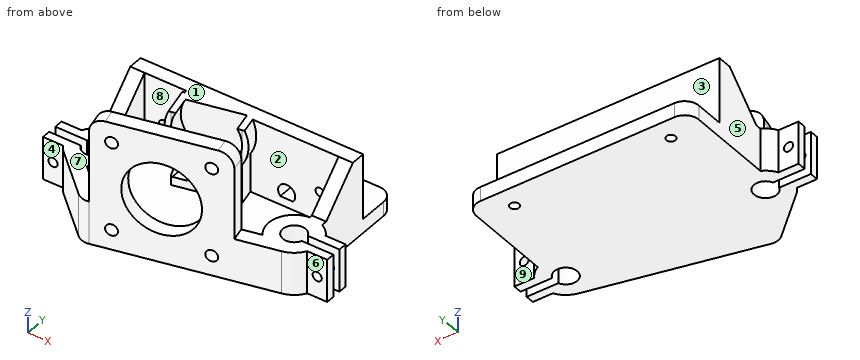
from build123d import *

# Parameters (mm, degrees)
BOSS_EXTRUDE1_DEPTH = 15
SKETCH2_R           = 1.6
CUT_EXTRUDE1_DEPTH  = 62.324670446
BOSS_EXTRUDE2_DEPTH = 30
FILLET1_R           = 5
CUT_EXTRUDE2_REACH  = 84.635
SKETCH4_R           = 12.5
SKETCH4_R_2         = 2
BOSS_EXTRUDE3_DEPTH = 2
BOSS_EXTRUDE4_DEPTH = 26
SKETCH7_W           = 78
SKETCH7_H           = 13
BOSS_EXTRUDE5_DEPTH = 5
BOSS_EXTRUDE6_DEPTH = 10
SKETCH9_R           = 11
CUT_EXTRUDE4_DEPTH  = 7
CHAMFER1_SIZE       = 13
SKETCH10_W          = 78
SKETCH10_H          = 5
BOSS_EXTRUDE7_DEPTH = 15
SKETCH11_R          = 1.6
CUT_EXTRUDE5_DEPTH  = 77.996527229
CUT_EXTRUDE6_REACH  = 85.597
SKETCH12_R          = 1.5
FILLET2_R           = 5
CUT_EXTRUDE7_REACH  = 85.597


with BuildPart() as part:
    # Sketch1 → Boss-Extrude1 (new body)
    with BuildSketch(Plane.XY):
        with BuildLine():
            Line((-39, 28), (39, 28))
            Line((39, 28), (39, 8.062257748))
            ThreePointArc((39, 8.062257748), (41.160225429, 6.561373535), (42.794228634, 4.5))
            Line((42.794228634, 4.5), (49.794228634, 4.5))
            Line((49.794228634, 4.5), (49.794228634, 1.5))
            Line((49.794228634, 1.5), (38.708099244, 1.5))
            ThreePointArc((38.708099244, 1.5), (31, 0), (38.708099244, -1.5))
            Line((38.708099244, -1.5), (49.794228634, -1.5))
            Line((49.794228634, -1.5), (49.794228634, -4.5))
            Line((49.794228634, -4.5), (42.794228634, -4.5))
            ThreePointArc((42.794228634, -4.5), (40.323053514, -7.257072501), (36.951023531, -8.785983564))
            Line((36.951023531, -8.785983564), (-23.82345919, -22.281620679))
            Line((-23.82345919, -22.281620679), (-41.045145267, -6.667549678))
            ThreePointArc((-41.045145267, -6.667549678), (-42.004044217, -5.651846124), (-42.794228634, -4.5))
            Line((-42.794228634, -4.5), (-49.794228634, -4.5))
            Line((-49.794228634, -4.5), (-49.794228634, -1.5))
            Line((-49.794228634, -1.5), (-38.708099244, -1.5))
            ThreePointArc((-38.708099244, -1.5), (-31, 0), (-38.708099244, 1.5))
            Line((-38.708099244, 1.5), (-49.794228634, 1.5))
            Line((-49.794228634, 1.5), (-49.794228634, 4.5))
            Line((-49.794228634, 4.5), (-42.794228634, 4.5))
            ThreePointArc((-42.794228634, 4.5), (-41.160225429, 6.561373535), (-39, 8.062257748))
            Line((-39, 8.062257748), (-39, 28))
        make_face()
        with BuildLine():
            Line((-34, 23), (34, 23))
            Line((34, 23), (34, 8.94427191))
            ThreePointArc((34, 8.94427191), (26.676479172, 3.423302649), (27.996581118, -5.652620982))
            Line((27.996581118, -5.652620982), (-22.38171768, -16.839672004))
            Line((-22.38171768, -16.839672004), (-31.713897446, -8.378635331))
            ThreePointArc((-31.713897446, -8.378635331), (-26.077363193, 1.177519599), (-34, 8.94427191))
            Line((-34, 8.94427191), (-34, 23))
        make_face(mode=Mode.SUBTRACT)
    extrude(amount=BOSS_EXTRUDE1_DEPTH)

    # Sketch2 → Cut-Extrude1 (cut, through all)
    with BuildSketch(Plane.XZ.offset(4.5)):
        with Locations((-46.294228634, 7.5)):
            Circle(SKETCH2_R)
        with Locations((46.294228634, 7.5)):
            Circle(SKETCH2_R)
    extrude(amount=-CUT_EXTRUDE1_DEPTH, mode=Mode.SUBTRACT)

    # Sketch3 → Boss-Extrude2 (add)
    with BuildSketch(Plane.XY.offset(15)):
        Polygon((-22.38171768, -16.839672004), (-21.297815718, -21.720773984), (22.6321021, -11.965656329), (21.548200138, -7.084554349), align=None)
    extrude(amount=BOSS_EXTRUDE2_DEPTH)

    # Fillet1
    fillet1_edges = [part.edges().sort_by_distance(p)[0] for p in [
        (-23.82345919, -22.281620679, 7.5),
        (22.090151119, -9.525105339, 45),
        (-21.839766699, -19.280222994, 45),
    ]]
    fillet(fillet1_edges, radius=FILLET1_R)

    # Sketch4 → Cut-Extrude2 (cut, up to next)
    with BuildSketch(Plane(origin=(3.595804379, -16.192873979, 0), x_dir=(0.9762203959642155, 0.21678039234089044, 0), z_dir=(0.21678039234089044, -0.9762203959642155, 0)), mode=Mode.PRIVATE) as cut_extrude2_sk1:
        with Locations((-3, 22.5)):
            Circle(SKETCH4_R)
    cut_extrude2_tool1 = extrude(cut_extrude2_sk1.sketch, amount=-CUT_EXTRUDE2_REACH, mode=Mode.PRIVATE) & part.part
    # Sketch4 → Cut-Extrude2 (cut, up to next)
    with BuildSketch(Plane(origin=(3.595804379, -16.192873979, 0), x_dir=(0.9762203959642155, 0.21678039234089044, 0), z_dir=(0.21678039234089044, -0.9762203959642155, 0)), mode=Mode.PRIVATE) as cut_extrude2_sk2:
        with Locations((-18.5, 38)):
            Circle(SKETCH4_R_2)
    cut_extrude2_tool2 = extrude(cut_extrude2_sk2.sketch, amount=-CUT_EXTRUDE2_REACH, mode=Mode.PRIVATE) & part.part
    # Sketch4 → Cut-Extrude2 (cut, up to next)
    with BuildSketch(Plane(origin=(3.595804379, -16.192873979, 0), x_dir=(0.9762203959642155, 0.21678039234089044, 0), z_dir=(0.21678039234089044, -0.9762203959642155, 0)), mode=Mode.PRIVATE) as cut_extrude2_sk3:
        with Locations((12.5, 38)):
            Circle(SKETCH4_R_2)
    cut_extrude2_tool3 = extrude(cut_extrude2_sk3.sketch, amount=-CUT_EXTRUDE2_REACH, mode=Mode.PRIVATE) & part.part
    # Sketch4 → Cut-Extrude2 (cut, up to next)
    with BuildSketch(Plane(origin=(3.595804379, -16.192873979, 0), x_dir=(0.9762203959642155, 0.21678039234089044, 0), z_dir=(0.21678039234089044, -0.9762203959642155, 0)), mode=Mode.PRIVATE) as cut_extrude2_sk4:
        with Locations((12.5, 7)):
            Circle(SKETCH4_R_2)
    cut_extrude2_tool4 = extrude(cut_extrude2_sk4.sketch, amount=-CUT_EXTRUDE2_REACH, mode=Mode.PRIVATE) & part.part
    # Sketch4 → Cut-Extrude2 (cut, up to next)
    with BuildSketch(Plane(origin=(3.595804379, -16.192873979, 0), x_dir=(0.9762203959642155, 0.21678039234089044, 0), z_dir=(0.21678039234089044, -0.9762203959642155, 0)), mode=Mode.PRIVATE) as cut_extrude2_sk5:
        with Locations((-18.5, 7)):
            Circle(SKETCH4_R_2)
    cut_extrude2_tool5 = extrude(cut_extrude2_sk5.sketch, amount=-CUT_EXTRUDE2_REACH, mode=Mode.PRIVATE) & part.part
    add(cut_extrude2_tool1.solids().sort_by_distance((0.667143, -16.843215, 22.5))[0], mode=Mode.SUBTRACT)
    add(cut_extrude2_tool2.solids().sort_by_distance((-14.464273, -20.203311, 38))[0], mode=Mode.SUBTRACT)
    add(cut_extrude2_tool3.solids().sort_by_distance((15.798559, -13.483119, 38))[0], mode=Mode.SUBTRACT)
    add(cut_extrude2_tool4.solids().sort_by_distance((15.798559, -13.483119, 7))[0], mode=Mode.SUBTRACT)
    add(cut_extrude2_tool5.solids().sort_by_distance((-14.464273, -20.203311, 7))[0], mode=Mode.SUBTRACT)

    # Sketch5 → Boss-Extrude3 (add)
    with BuildSketch(Plane(origin=(0, 0, 0), x_dir=(-1, 0, 0), z_dir=(0, 0, -1))):
        Polygon((-34, 23), (-34, 8.94427191), (-27.996581118, -5.652620982), (22.38171768, -16.839672004), (31.713897446, -8.378635331), (29.251891486, 2.846497001), (34, 8.94427191), (34, 23), align=None)
    extrude(amount=-BOSS_EXTRUDE3_DEPTH)

    # Sketch6 → Boss-Extrude4 (add)
    with BuildSketch(Plane.XY.offset(2)):
        Polygon((3.087469785, 23), (4.388152139, 17.142677624), (-17.088696572, 12.373508993), (-19.448424866, 23), align=None)
    extrude(amount=BOSS_EXTRUDE4_DEPTH)

    # Sketch7 → Boss-Extrude5 (add)
    with BuildSketch(Plane(origin=(0, 23, 0), x_dir=(1, 0, 0), z_dir=(0, 1, 0))):
        with Locations((0, -21.5)):
            Rectangle(SKETCH7_W, SKETCH7_H)
    extrude(amount=BOSS_EXTRUDE5_DEPTH)

    # Sketch8 → Boss-Extrude6 (add)
    with BuildSketch(Plane(origin=(-3.421611029, 15.408434485, 0), x_dir=(0.9762203959642155, 0.21678039234089055, 0), z_dir=(0.21678039234089053, -0.9762203959642154, 0))):
        with BuildLine():
            Line((-14.779218989, 28), (-12.526279442, 28))
            ThreePointArc((-12.526279442, 28), (-3, 11.5), (6.526279442, 28))
            Line((6.526279442, 28), (8.779218989, 28))
            ThreePointArc((8.779218989, 28), (-3, 9.5), (-14.779218989, 28))
        make_face()
    extrude(amount=-BOSS_EXTRUDE6_DEPTH)

    # Sketch9 → Cut-Extrude4 (cut)
    with BuildSketch(Plane(origin=(-3.421611029, 15.408434485, 0), x_dir=(0.9762203959642155, 0.21678039234089055, 0), z_dir=(0.21678039234089053, -0.9762203959642154, 0))):
        with Locations((-3, 22.5)):
            Circle(SKETCH9_R)
    extrude(amount=-CUT_EXTRUDE4_DEPTH, mode=Mode.SUBTRACT)

    # Chamfer1
    chamfer1_edges = [part.edges().sort_by_distance(p)[0] for p in [
        (-36.5, 23, 15),
        (36.5, 23, 15),
    ]]
    chamfer(chamfer1_edges, length=CHAMFER1_SIZE - 0.0001)  # a hair under: the kernel refuses the full size

    # Sketch10 → Boss-Extrude7 (add)
    with BuildSketch(Plane(origin=(0, 28, 0), x_dir=(1, 0, 0), z_dir=(0, 1, 0))):
        with Locations((0, -2.5)):
            Rectangle(SKETCH10_W, SKETCH10_H)
    extrude(amount=BOSS_EXTRUDE7_DEPTH)

    # Sketch11 → Cut-Extrude5 (cut, through all)
    with BuildSketch(Plane.XY.offset(5)):
        with Locations((-27.4, 35.5)):
            Circle(SKETCH11_R)
        with Locations((27.4, 35.5)):
            Circle(SKETCH11_R)
    extrude(amount=-CUT_EXTRUDE5_DEPTH, mode=Mode.SUBTRACT)

    # Sketch12 → Cut-Extrude6 (cut, up to next)
    with BuildSketch(Plane(origin=(0, 28, 0), x_dir=(1, 0, 0), z_dir=(0, 1, 0)), mode=Mode.PRIVATE) as cut_extrude6_sk1:
        with Locations(Location((27.4, -12.5, 0), (0, 0, 270))):
            Circle(SKETCH12_R)
    cut_extrude6_tool1 = extrude(cut_extrude6_sk1.sketch, amount=-CUT_EXTRUDE6_REACH, mode=Mode.PRIVATE) & part.part
    # Sketch12 → Cut-Extrude6 (cut, up to next)
    with BuildSketch(Plane(origin=(0, 28, 0), x_dir=(1, 0, 0), z_dir=(0, 1, 0)), mode=Mode.PRIVATE) as cut_extrude6_sk2:
        with Locations(Location((-27.4, -12.5, 0), (0, 0, 270))):
            Circle(SKETCH12_R)
    cut_extrude6_tool2 = extrude(cut_extrude6_sk2.sketch, amount=-CUT_EXTRUDE6_REACH, mode=Mode.PRIVATE) & part.part
    add(cut_extrude6_tool1.solids().sort_by_distance((27.4, 28, 12.5))[0], mode=Mode.SUBTRACT)
    add(cut_extrude6_tool2.solids().sort_by_distance((-27.4, 28, 12.5))[0], mode=Mode.SUBTRACT)

    # Fillet2
    fillet2_edges = [part.edges().sort_by_distance(p)[0] for p in [
        (-39, 43, 2.5),
        (39, 43, 2.5),
    ]]
    fillet(fillet2_edges, radius=FILLET2_R)

    # Sketch14 → Cut-Extrude7 (cut, up to next)
    with BuildSketch(Plane(origin=(0, 28, 0), x_dir=(1, 0, 0), z_dir=(0, 1, 0)), mode=Mode.PRIVATE) as cut_extrude7_sk1:
        with BuildLine():
            Line((18.034627306, -5), (13.562491351, -5))
            ThreePointArc((13.562491351, -5), (15.798559328, -10), (18.034627306, -5))
        make_face()
    cut_extrude7_tool1 = extrude(cut_extrude7_sk1.sketch, amount=-CUT_EXTRUDE7_REACH, mode=Mode.PRIVATE) & part.part
    # Sketch14 → Cut-Extrude7 (cut, up to next)
    with BuildSketch(Plane(origin=(0, 28, 0), x_dir=(1, 0, 0), z_dir=(0, 1, 0)), mode=Mode.PRIVATE) as cut_extrude7_sk2:
        with BuildLine():
            Line((-12.228204969, -5), (-16.700340924, -5))
            ThreePointArc((-16.700340924, -5), (-14.464272947, -10), (-12.228204969, -5))
        make_face()
    cut_extrude7_tool2 = extrude(cut_extrude7_sk2.sketch, amount=-CUT_EXTRUDE7_REACH, mode=Mode.PRIVATE) & part.part
    add(cut_extrude7_tool1.solids().sort_by_distance((15.798559, 28, 7.296048))[0], mode=Mode.SUBTRACT)
    add(cut_extrude7_tool2.solids().sort_by_distance((-14.464273, 28, 7.296048))[0], mode=Mode.SUBTRACT)


solid = part.part
Can you work these out from the model? Positions are in its coordinate system, mm. Face numbers are marked on the shaded views. A direction names the side the tool comes from. Coordinates: 2 decimals unless noted, no trailing zeros. Write each loop counter-clockwise with the first axis right and the second up, starting at its lowest first coordinate (ties: lowest second). Pieces come first, ordered by that corner, then holes.
Q1. For P1, Ø12, axis at x = -42.5, z = 10, coming from the +Y side; P2, Ø4, axis at x = -46.29, z = 7.5, coming from the -Y side; P3, Ø3.5, axis at x = -14.46, z = 7, coming from the +Y side; P4, Ø12, axis at x = -33, z = 40.5, coming from the +Y side, each with a flat end and sliding along its axis, tell me the tip position at first contact or that it passes through.
Results found:
P1: stops at y = 28
P2: stops at y = -4.5
P3: stops at y = -14.69
P4: passes through
Q2. Which directions (+Z, -Z, +X, -X, +Y, -Y) give clear straight access to the entire face, cutting with the end or side of a thin tool? Please do the marked faces 5, 6, 7, 8 and 9.
Results found:
face 5: +Z, -Z, -X, +Y
face 6: +Z, -Z, +X, -Y
face 7: +Z, -X, -Y
face 8: +Z
face 9: +Z, -Z, +X, +Y
Q3. Imagine slicing it at B-B, the plane x = 40.5. List the corners of the cut face in (y, z) for me, plus the area to 3 significant figures.
Results found:
outline: (-7.12, 0) - (-1.5, 0) - (-1.5, 15) - (-7.12, 15) - close; (1.5, 0) - (7.12, 0) - (7.12, 15) - (1.5, 15) - close
area: 169 mm2
Q4. Imagine slicing it at D-D, the plane z = 20.5. List the corners of the cut face in (x, y) for me, plus the area to 3 significant figures.
Results found:
outline: (-39, 15.5) - (-34, 15.5) - (-34, 23) - (-19.45, 23) - (-19.26, 22.14) - (-21.06, 21.74) - (-18.89, 11.97) - (-16.91, 12.41) - (-18.43, 19.25) - (2.69, 23.94) - (4.21, 17.1) - (6.19, 17.54) - (4.98, 23) - (34, 23) - (34, 15.5) - (39, 15.5) - (39, 28) - (-39, 28) - close; (-22.38, -16.84) - (-21.3, -21.72) - (-11.38, -19.52) - (-12.46, -14.64) - close; (11.63, -9.29) - (12.71, -14.17) - (22.63, -11.97) - (21.55, -7.08) - close
area: 630 mm2
Q5. Imagine slicing it at A-A, the plane y = 35.5. List the corners of the cut face in (x, z) for me.
Results found:
outline: (-39, 0) - (-29, 0) - (-29, 5) - (-39, 5) - close; (-25.8, 0) - (25.8, 0) - (25.8, 5) - (-25.8, 5) - close; (29, 0) - (39, 0) - (39, 5) - (29, 5) - close
Q6. If we mould it in two halves opening along Y, with no side actions, what happens to the marked faces 1, 2, 3 and 4? For each: +Y half, -Y half, draft (parallel to the pull), parting line (faces both ways), or undercut.
Results found:
face 1: draft
face 2: undercut
face 3: +Y half
face 4: -Y half
Q7. Imagine slicing it at C-C, the plane y = 0. List the corners of the cut face in (x, z) for me.
Results found:
outline: (-31, 0) - (31, 0) - (31, 15) - (26, 15) - (26, 2) - (-26, 2) - (-26, 15) - (-31, 15) - close
Q8. Please list where these lines run through material, in increasing order: L1, parallel to X at y = 3, z = 7; L2, parallel to X at y = -3, z = 11; L3, parallel to Z at x = -21, y = 27.
Results found:
L1: x = -49.79 to -47.81, -44.77 to -37.65, -32.35 to -26.51, 26.51 to 32.35, 37.65 to 44.77, 47.81 to 49.79
L2: x = -49.79 to -37.65, -32.35 to -26.51, 26.51 to 32.35, 37.65 to 49.79
L3: z = 0 to 28
